from build123d import *

# Parameters (mm, degrees)
SKETCH_W        = 15
SKETCH_H        = 150
SKETCH_R        = 3.45
PAD_DEPTH       = 12
SKETCH003_W     = 10
SKETCH003_H     = 4
SKETCH003_W_2   = 6
POCKET002_DEPTH = 15.001
SKETCH004_R     = 20
POCKET003_DEPTH = 150.001
FILLET_R        = 2


with BuildPart() as part:
    # Sketch → Pad (new body)
    with BuildSketch(Plane.XY):
        with Locations((7.5, 75)):
            Rectangle(SKETCH_W, SKETCH_H)
        with Locations((7.5, 138)):
            Circle(SKETCH_R, mode=Mode.SUBTRACT)
        with Locations((7.5, 75)):
            Circle(SKETCH_R, mode=Mode.SUBTRACT)
        with Locations((7.5, 12)):
            Circle(SKETCH_R, mode=Mode.SUBTRACT)
    extrude(amount=PAD_DEPTH)

    # Sketch003 → Pocket002 (cut, through all)
    with BuildSketch(Plane.YZ):
        with Locations((30, 2)):
            Rectangle(SKETCH003_W, SKETCH003_H)
        with Locations((57, 2)):
            Rectangle(SKETCH003_W_2, SKETCH003_H)
        with Locations((120, 2)):
            Rectangle(SKETCH003_W, SKETCH003_H)
        with Locations((93, 2)):
            Rectangle(SKETCH003_W_2, SKETCH003_H)
    extrude(amount=POCKET002_DEPTH, mode=Mode.SUBTRACT)

    # Sketch004 → Pocket003 (cut, through all)
    with BuildSketch(Plane.XZ):
        with Locations((7.5, 30.540496)):
            Circle(SKETCH004_R)
    extrude(amount=-POCKET003_DEPTH, mode=Mode.SUBTRACT)

    # Fillet
    fillet_edges = [part.edges().sort_by_distance(p)[0] for p in [
        (15, 25, 2),
        (15, 30, 4),
        (15, 35, 2),
        (15, 12.5, 0),
        (7.5, 25, 0),
        (7.5, 35, 0),
        (0, 12.5, 0),
        (0, 25, 2),
        (0, 30, 4),
        (0, 35, 2),
        (0, 44.5, 0),
        (15, 44.5, 0),
        (7.5, 0, 0),
        (0, 0, 6),
        (15, 0, 6),
        (0, 75, 0),
        (15, 75, 0),
        (15, 105.5, 0),
        (0, 105.5, 0),
        (0, 137.5, 0),
        (15, 137.5, 0),
        (0, 150, 6),
        (7.5, 150, 0),
        (15, 150, 6),
        (15, 54, 2),
        (15, 57, 4),
        (15, 60, 2),
        (15, 90, 2),
        (15, 93, 4),
        (15, 96, 2),
        (15, 115, 2),
        (15, 120, 4),
        (15, 125, 2),
        (7.5, 54, 0),
        (7.5, 60, 0),
        (0, 54, 2),
        (0, 57, 4),
        (0, 60, 2),
        (7.5, 90, 0),
        (7.5, 96, 0),
        (0, 93, 4),
        (0, 96, 2),
        (0, 90, 2),
        (7.5, 115, 0),
        (7.5, 125, 0),
        (0, 125, 2),
        (0, 120, 4),
        (0, 115, 2),
    ]]
    fillet(fillet_edges, radius=FILLET_R)


solid = part.part
Verification items for the finished model (mm, model axes). A direction names the side the tool comes from. Coordinates: 2 decimals unless noted, no trailing zeros. Order: outer loops, then holes, each group sorted by start corner. A loop starts at its lowest first (then second) coordinate and runs counter-clockwise, first axis right, second up.
1. Scan lines: line 1 (Y direction, x = 11, z = 2); line 2 (Y direction, x = 7.5, z = 6.75); line 3 (X direction, y = 138, z = 3.25). Record each from-to range of solid material in increasing order.
Results found:
line 1: y = 0 to 25, 35 to 54, 60 to 90, 96 to 115, 125 to 150
line 2: y = 0 to 8.55, 15.45 to 71.55, 78.45 to 134.55, 141.45 to 150
line 3: x = 0 to 4.05, 10.95 to 15
2. Set-up check for faces 1 (the face through (7, 150, 7)), 2 (the face through (7, 93, 4)): record each of +Z, -Z, +X, -X, +Y, -Y from which the full face is reachable in a straight line by a thin tool's end or side.
Results found:
face 1: +Z, -Z, +X, -X, +Y
face 2: -Z, +X, -X
3. Sectioned sample at B-B, the plane y = 92.5. Record the cut outline in (x, z).
Results found:
outline: (0, 6) arc R2 ccw to (2, 4) - (13, 4) arc R2 ccw to (15, 6) - (15, 12) arc R20 cw to (0, 12) - close
4. Sectioned sample at A-A, the plane y = 12. Record the cut outline in (x, z).
Results found:
outline: (0, 2) arc R2 ccw to (2, 0) - (4.05, 0) - (4.05, 10.84) arc R20 cw to (0, 12) - close; (10.95, 0) - (13, 0) arc R2 ccw to (15, 2) - (15, 12) arc R20 cw to (10.95, 10.84) - close
5. Sectioned sample at C-C, the plane x = 6. Give the number of separate pieces and of enclosed holes in the cut face, and give its area (3 significant figures).
Results found:
separate pieces: 4
enclosed holes: 0
area: 1,260 mm2
6. Release check for a two-part mould opening along X. For faces 3 (the face through (7, 45, 0)), 4 (the face through (15, 74, 8)), 5 (the face through (0, 74, 8)), 6 (the face through (7.05, 141.42, 5.35)) record: +X half, -X half, draft (parallel to the pull), parting line (faces both ways), or undercut.
Results found:
face 3: draft
face 4: +X half
face 5: -X half
face 6: undercut
7. Sectioned sample at D-D, the plane y = 77. Record the cut outline in (x, z).
Results found:
outline: (0, 2) arc R2 ccw to (2, 0) - (4.69, 0) - (4.69, 10.74) arc R20 cw to (0, 12) - close; (10.31, 0) - (13, 0) arc R2 ccw to (15, 2) - (15, 12) arc R20 cw to (10.31, 10.74) - close
8. Go/stop test with flat-tipped pins: pin 1 Ø5.5 at (x, y) = (7.5, 138) entering from -Z; pin 2 Ø1 at (y, z) = (125.5, 4.5) entering from +X; pin 3 Ø6.5 at (x, y) = (5, 93.5) entering from -Z; pin 4 Ø5 at (x, y) = (9, 58.5) entering from -Z. Record where each tip stops, or that it passes through.
Results found:
pin 1: passes through
pin 2: stops at x = 14.73
pin 3: stops at z = 0.44
pin 4: stops at z = 0.27
